```python
from build123d import *

# Parameters (mm, degrees)
SKETCH3_R           = 1.7145
BOSS_EXTRUDE1_DEPTH = 3.048
FILLET2_R           = 0.508


with BuildPart() as part:
    # Sketch2 → Revolve1 (revolve)
    with BuildSketch(Plane.XY, mode=Mode.PRIVATE) as revolve1_sk:
        Polygon((0, 0), (15.113, 0), (15.113, 19.177), (1.905, 19.177), (1.905, 16.637), (0, 16.637), align=None)
    revolve(revolve1_sk.sketch.rotate(Axis((0, 0, 0), (0, 1, 0)), 90), axis=Axis((0, 0, 0), (0, 1, 0)))

    # Sketch3 → Boss-Extrude1 (add)
    with BuildSketch(Plane.XZ):
        with BuildLine():
            Line((-19.05, 4.445), (19.05, 4.445))
            ThreePointArc((19.05, 4.445), (23.495, 0), (19.05, -4.445))
            Line((19.05, -4.445), (-19.05, -4.445))
            ThreePointArc((-19.05, -4.445), (-23.495, 0), (-19.05, 4.445))
        make_face()
        with Locations(Location((19.05, 0, 0), (0, 0, 270))):
            Circle(SKETCH3_R, mode=Mode.SUBTRACT)
        with Locations(Location((-19.05, 0, 0), (0, 0, 270))):
            Circle(SKETCH3_R, mode=Mode.SUBTRACT)
    extrude(amount=-BOSS_EXTRUDE1_DEPTH)

    # Fillet2
    fillet2_edges = [part.edges().sort_by_distance(p)[0] for p in [
        (0, 19.177, 15.113),
    ]]
    fillet(fillet2_edges, radius=FILLET2_R)


solid = part.part
```
Verification items for the finished model (mm, model axes). A direction names the side the tool comes from. Coordinates: 2 decimals unless noted, no trailing zeros. Write each loop counter-clockwise with the first axis right and the second up, starting at its lowest first coordinate (ties: lowest second). Pieces come first, ordered by that corner, then holes. Notation, with made-up numbers: M 74,45 L 90,45 A11 cw 90,56 Z; hole C -10.5,28 d11. An arc over 180 degrees is marked long. One line per item, written item: value.
Item 1: Section check B-B, the plane x = 0. Record the boundary of the cut face in (y, z) (3 decimals).
Check sheet entries:
outline: M 0,-15.113 L 18.669,-15.113 A0.508 ccw 19.177,-14.605 L 19.177,-1.905 L 16.637,-1.905 L 16.637,1.905 L 19.177,1.905 L 19.177,14.605 A0.508 ccw 18.669,15.113 L 0,15.113 Z
Item 2: Mould release check, pull along X, two halves, no side actions. Record for faces 4 (the cylindrical face through (-17.35, 1.5, 0.22)), 5 (the flat face through (17, 2, -4.445)), 6 (the cylindrical face through (-23.494, 1.503, -0.098)), 7 (the cylindrical face through (23.494, 1.503, 0.098)): pulls with the +X half, pulls with the -X half, needs draft (parallel to the pull), parting line crosses it, or undercut.
Check sheet entries:
face 4: undercut
face 5: needs draft
face 6: pulls with the -X half
face 7: pulls with the +X half
Item 3: Scan lines: line 1 along X through (y, z) = (2.45, 0) (1 decimal); line 2 along X through (y, z) = (17.65, 0) (3 decimals); line 3 along Y through (x, z) = (-8.5, 12). Record each from-to range of solid material in increasing order.
Check sheet entries:
line 1: x = -23.5 to -20.8, -17.3 to 17.3, 20.8 to 23.5
line 2: x = -15.113 to -1.905, 1.905 to 15.113
line 3: y = 0 to 19.17
Item 4: Gauge pin test, flat ends, axial feed: pin 1 Ø1.5 at (y, z) = (9, 6.5) entering from -X; pin 2 Ø0.9 at (x, y) = (-18, 1.5) entering from -Z (3 decimals); pin 3 Ø6 at (x, y) = (12, 10) entering from -Z; pin 4 Ø4.5 at (x, z) = (0, 0) entering from -Y. Record the tip position at first contact, or that the pin passes through.
Check sheet entries:
pin 1: stops at x = -13.98
pin 2: stops at z = -4.445
pin 3: stops at z = -12.14
pin 4: stops at y = 0
Item 5: Section check C-C, the plane x = 20. Record the boundary of the cut face in (y, z).
Check sheet entries:
outline: M 0,-4.34 L 3.05,-4.34 L 3.05,-1.43 L 0,-1.43 Z; M 0,1.43 L 3.05,1.43 L 3.05,4.34 L 0,4.34 Z
Item 6: Section check A-A, the plane z = 0. Record the boundary of the cut face in (x, y) (1 decimal), plus the area to 3 significant figures.
Check sheet entries:
outline: M -23.5,0 L -20.8,0 L -20.8,3 L -23.5,3 Z; M -17.3,0 L 17.3,0 L 17.3,3 L 15.1,3 L 15.1,18.7 A0.5 ccw 14.6,19.2 L 1.9,19.2 L 1.9,16.6 L -1.9,16.6 L -1.9,19.2 L -14.6,19.2 A0.5 ccw -15.1,18.7 L -15.1,3 L -17.3,3 Z; M 20.8,0 L 23.5,0 L 23.5,3 L 20.8,3 Z
area: 600 mm^2
Item 7: Section check D-D, the plane y = 9. Record the boundary of the cut face in (x, z), plus the area to 3 significant figures.
Check sheet entries:
outline: C 0,0 d30.23
area: 718 mm^2
Item 8: Access from +Z, -Z, +X, -X, +Y, -Y to the whole of each face (thin tool, end or side, straight path). Record for faces 1 (the flat face through (17, 2, 4.445)), 2 (the flat face through (0, 16.637, 0)), 3 (the flat face through (-17, 2, 4.445)).
Check sheet entries:
face 1: +Z, +X, +Y, -Y
face 2: +Y
face 3: +Z, -X, +Y, -Y
